Drawing for the job (mm, zero at the part's lowest x, y, z). Coordinates: 2 decimals unless noted, no trailing zeros. Loops run counter-clockwise (first coordinate to the right, second up) from the corner with the lowest first, then second, coordinate; pieces in that order, holes last. Notation, with made-up numbers: (8, -6) -> (61, -6) arc R24 cw to (61, 10) -> close; hole circle Ø7 at (-15.75, 20.25). An arc over 180 degrees is marked (long way). Write each question's results on one line, items separated by ' | '.
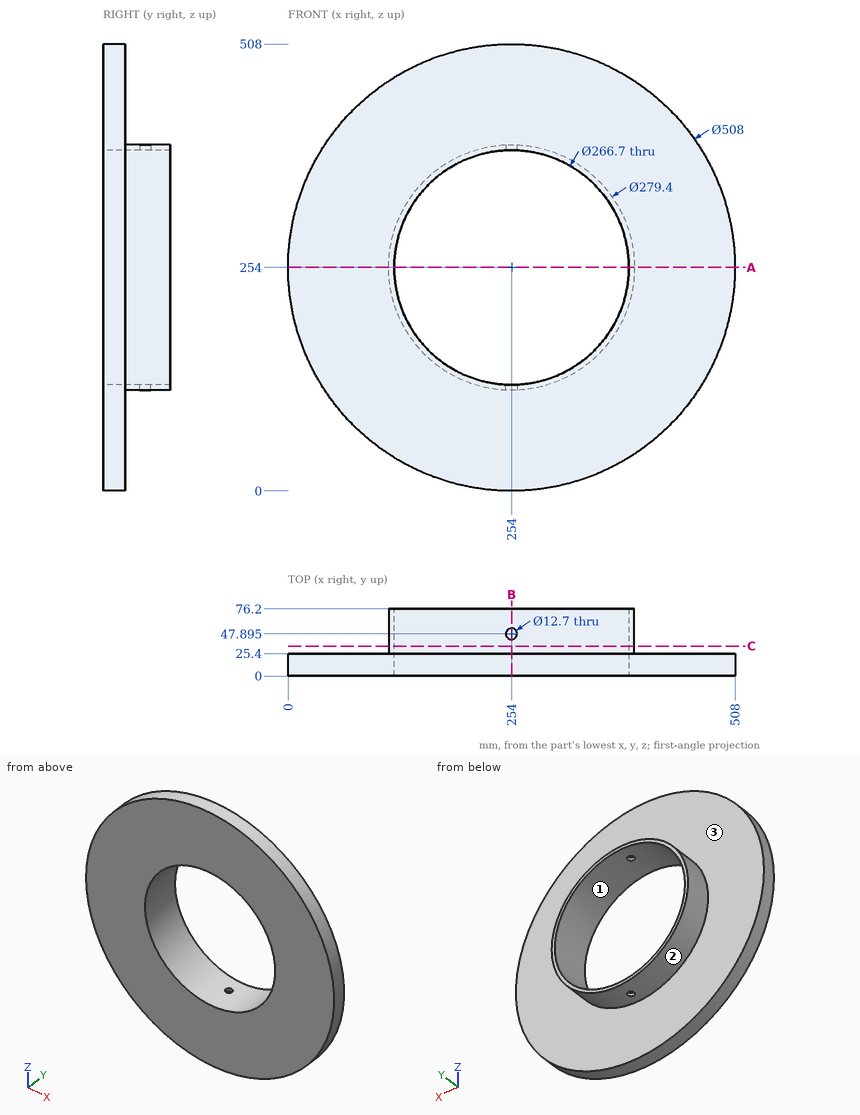
1) Two-plate mould, pull along Z, no slides. Class the marked faces 1, 2 and 3: pulls with the +Z half, pulls with the -Z half, needs draft (parallel to the pull), parting line crosses it, or undercut.
Outcome:
face 1: undercut | face 2: parting line crosses it | face 3: needs draft
2) Slice it at B-B (x = 254). Count the separate pieces of the cut face and the enclosed holes in it, then the cut area to 3 significant figures.
Outcome:
separate pieces: 4 | enclosed holes: 0 | area: 6,610 mm^2
3) Pin check, flat tips, straight feed: pin 1 (10 mm diameter, centred on x = 151.5, y = 64, fed in from -Z); pin 2 (3 mm diameter, centred on x = 370.5, y = 21.5, fed in from -Z) (1 decimal); pin 3 (4 mm diameter, centred on y = 56, z = 334.5, fed in from +X). Stop position of each tip, or through.
Outcome:
pin 1: stops at z = 153.95 | pin 2: stops at z = 27.5 | pin 3: stops at x = 369.56
4) Slice it at C-C (y = 34). Write the cut outline in (x, z), then the cut area to 3 significant figures.
Outcome:
outline: circle Ø279.4 at (254, 254); hole circle Ø266.7 at (254, 254) | area: 5,450 mm^2
5) Drill centre lines: L1, parallel to Y at x = 254, z = 118 (1 decimal); L2, parallel to Y at x = 456, z = 166.5; L3, parallel to X at y = 62, z = 152 (1 decimal). Where is each one in solid material? Low to high. Write a range as from..to.
Outcome:
L1: y = 0..41.5, 54.2..76.2 | L2: y = 0..25.4 | L3: x = 158.5..168.1, 339.9..349.5
6) Slice it at A-A (z = 254). Write the cut outline in (x, y).
Outcome:
outline: (0, 0) -> (120.65, 0) -> (120.65, 76.2) -> (114.3, 76.2) -> (114.3, 25.4) -> (0, 25.4) -> close; (387.35, 0) -> (508, 0) -> (508, 25.4) -> (393.7, 25.4) -> (393.7, 76.2) -> (387.35, 76.2) -> close
